CAD build for the part. Positions are in the model's coordinates, mm. A direction names the side the tool comes from. Give positions to 0.01 mm unless a question says otherwise; leave off trailing zeros. Loops run counter-clockwise (first coordinate to the right, second up) from the corner with the lowest first, then second, coordinate; pieces in that order, holes last.
Autodesk Inventor part; units mm, degrees
ref_plane "YZ Plane" through (0, 0, 0) normal (1, 0, 0) x (0, 1, 0)
ref_plane "XZ Plane" through (0, 0, 0) normal (0, 1, 0) x (-1, 0, 0)
ref_plane "XY Plane" through (0, 0, 0) normal (0, 0, 1) x (1, 0, 0)
sketch "Skizze1" plane through (0, 0, 0) normal (0, 0, 1) x (1, 0, 0)
  circle A0 centre (5, 33) radius 4.25
  circle A1 centre (37.5, 5) radius 4.25
  circle A2 centre (70, 23) radius 4.25
  circle A3 centre (70, 5) radius 4.25
  circle A4 centre (5, 33) radius 2
  circle A5 centre (37.5, 5) radius 2
  circle A6 centre (70, 5) radius 2
  circle A7 centre (70, 23) radius 2
  point P0 (0, 0)
  dimension "d0" = 8.5
  dimension "d1" = 33
  dimension "d2" = 5
  dimension "d3" = 8.5
  dimension "d4" = 5
  dimension "d5" = 37.5
  dimension "d6" = 8.5
  dimension "d7" = 70
  dimension "d8" = 23
  dimension "d9" = 8.5
  dimension "d10" = 70
  dimension "d11" = 5
  dimension "d12" = 4
  dimension "d13" = 4
  dimension "d14" = 4
  dimension "d15" = 4
extrude "Extrusion1" add sketch "Skizze1" against normal blind 8
sketch "Skizze2" plane through (70, 23, -8) normal (0, 0, -1) x (-1, 0, 0)
  circle A0 centre (0, 0) radius 2
  circle A1 centre (0, 0) radius 4.25
  circle A2 centre (0, 0) radius 2
  circle A3 centre (0, -18) radius 4.25
  circle A4 centre (0, -18) radius 2
  circle A5 centre (32.5, -18) radius 4.25
  circle A6 centre (32.5, -18) radius 2
  circle A7 centre (65, 10) radius 4.25
  circle A8 centre (65, 10) radius 2
  line L0 (0, 0) -> (0, -18) construction
  line L1 (-4.25, 0) -> (-4.25, -18)
  line L2 (4.25, -18) -> (4.25, 0)
  arc A9 (4.25, 0) -> (-4.25, 0) centre (0, 0) ccw
  arc A10 (-4.25, -18) -> (4.25, -18) centre (0, -18) ccw
  line L3 (0, -18) -> (32.5, -18) construction
  line L4 (0, -22.25) -> (32.5, -22.25)
  line L5 (32.5, -13.75) -> (0, -13.75)
  arc A11 (0, -13.75) -> (0, -22.25) centre (0, -18) ccw
  arc A12 (32.5, -22.25) -> (32.5, -13.75) centre (32.5, -18) ccw
  circle A13 centre (32.5, -18) radius 2
  line L6 (65, 10) -> (32.5, -18) construction
  line L7 (62.226, 13.2198) -> (29.726, -14.7802)
  line L8 (35.274, -21.2198) -> (67.774, 6.7802)
  arc A14 (67.774, 6.7802) -> (62.226, 13.2198) centre (65, 10) ccw
  arc A15 (29.726, -14.7802) -> (35.274, -21.2198) centre (32.5, -18) ccw
  line L9 (0, 0) -> (32.5, -18) construction
  line L10 (-2.0591, -3.7179) -> (30.4409, -21.7179)
  line L11 (34.5591, -14.2821) -> (2.0591, 3.7179)
  arc A16 (2.0591, 3.7179) -> (-2.0591, -3.7179) centre (0, 0) ccw
  arc A17 (30.4409, -21.7179) -> (34.5591, -14.2821) centre (32.5, -18) ccw
  line L12 (0, 0) -> (65, 10) construction
  line L13 (0.6462, -4.2006) -> (65.6462, 5.7994)
  line L14 (64.3538, 14.2006) -> (-0.6462, 4.2006)
  arc A18 (-0.6462, 4.2006) -> (0.6462, -4.2006) centre (0, 0) ccw
  arc A19 (65.6462, 5.7994) -> (64.3538, 14.2006) centre (65, 10) ccw
  point P0 (70, -23)
  point P1 (0, -9)
  point P2 (16.25, -18)
  point P3 (48.75, -4)
  point P4 (16.25, -9)
  point P5 (32.5, 5)
  point P6 (50.9971, 3.5457)
  point P7 (31.9691, -12.8477)
  point P8 (12.9411, -2.3091)
  point P9 (-4.25, 0)
  point P10 (-4.25, -18)
  point P11 (4.25, -13.75)
  point P12 (4.25, -7.2121)
  point P13 (16.0545, -13.75)
extrude "Extrusion2" add sketch "Skizze2" against normal blind 2 contours A0 | L2 L13 A1 | A1 L11 L13 L2 | A1 L14 A7 L7 L13 L11 | L13 L2 L10 A1 | L13 L11 L7 L5 L10 L2 | L10 L2 L5 A3 L1 A1 | L11 A5 L5 L7 | L7 L13 A7 L8 A5 L11 | L7 A7 L13 | L5 L10 A5 L4 A3 L2 | L2 A3 L5 | L5 L7 A5 L10 | L5 A5 L7 | A4 | A6 | A8
fillet "Rundung1" radius 1 6 edges at (19.0029, 26.5457, -7) (38.0309, 10.1523, -7) (57.0589, 20.6909, -7) (53.9455, 9.25, -7) (65.75, 9.25, -7) (65.75, 15.7879, -7)
properties part number "200_Frame_Internal"
1. Saw through at A-A, the plane z = -4.75. List the corners of the cut face in (x, y), and give its area (3 significant figures).
Responses:
outline: circle Ø8.5 at (5, 33); circle Ø8.5 at (37.5, 5); circle Ø8.5 at (70, 5); circle Ø8.5 at (70, 23); hole circle Ø4 at (5, 33); hole circle Ø4 at (37.5, 5); hole circle Ø4 at (70, 5); hole circle Ø4 at (70, 23)
area: 177 mm2
2. Probe line 1 along X through (y, z) = (5, -5); line 2 along Y through (x, z) = (70, -3.15); line 3 along X through (y, z) = (4, -2.5). List the from-to ranges inside material, lowest first.
Responses:
line 1: x = 33.25 to 35.5, 39.5 to 41.75, 65.75 to 68, 72 to 74.25
line 2: y = 0.75 to 3, 7 to 9.25, 18.75 to 21, 25 to 27.25
line 3: x = 33.37 to 35.77, 39.23 to 41.63, 65.87 to 68.27, 71.73 to 74.13
3. Saw through at C-C, the plane x = 41. List the corners of the cut face in (y, z).
Responses:
outline: (0.75, -8) - (11.8, -8) - (11.8, -6) - (7.41, -6) - (7.41, 0) - (2.59, 0) - (2.59, -6) - (0.75, -6) - close; (23.16, -8) - (31.76, -8) - (31.76, -6) - (23.16, -6) - close
4. Tool access for faces 5 (the face through (5, 31, -3)), 6 (the face through (55, 20.31, -6.99)), 7 (the face through (7, 32, 0)): list every direction of +Z, -Z, +X, -X, +Y, -Y with a clear straight run to the whole face (end or side of a thin tool).
Responses:
face 5: +Z
face 6: +Z, -Z
face 7: +Z, +X, -X, +Y, -Y
5. Pull direction Y, two halves, no side cores. Call faces 1 (the face through (56.84, 10.02, -6.99)), 2 (the face through (74.25, 14, -7)), 3 (the face through (37.69, 32.27, -7.01)), 4 (the face through (46.46, 14.82, -7.01)): released by +Y, released by -Y, zero draft, split by the parting line, or undercut.
Responses:
face 1: undercut
face 2: zero draft
face 3: released by +Y
face 4: undercut
6. Drop flat-ended pins along their axis: pin 1 (4 mm diameter, centred on x = 44.5, z = -2.5, fed in from +Y); pin 2 (12 mm diameter, centred on x = 41, y = 30, fed in from +Z); pin 3 (0.6 mm diameter, centred on y = 13, z = -7.5, fed in from -X); pin 4 (1.5 mm diameter, centred on x = 38.5, z = -3, fed in from +Y). Give the stop position or say it passes through.
Responses:
pin 1: passes through
pin 2: stops at z = -6
pin 3: stops at x = 21.35
pin 4: stops at y = 9.24
7. Saw through at B-B, the plane y = 12. List the corners of the cut face in (x, z).
Responses:
outline: (22.86, -8) - (35.89, -8) - (35.89, -6) - (22.86, -6) - close; (41.37, -8) - (58.91, -8) - (58.91, -6) - (41.37, -6) - close; (65.75, -8) - (74.25, -8) - (74.25, -6) - (65.75, -6) - close
